Design review of the part built by this model. Coordinates are the model's own, in mm. Give positions to 0.01 mm unless a question says otherwise; leave off trailing zeros. Loops run counter-clockwise (first coordinate to the right, second up) from the corner with the lowest first, then second, coordinate; pieces in that order, holes last. Notation, with made-up numbers: (77.25, 67.5) -> (85.25, 67.5) arc R8 ccw to (85.25, 75.5) -> close; hole circle Ø10 at (-25.75, 69). An arc over 180 degrees is marked (long way). Answer in a Markdown table with one row per item. Add a question column.
(1) Consider section A-A on y = 153.5. Write out the cut boundary in (x, z), then the cut area to 3 significant figures.
(2) For pin 1 (1.2 mm diameter, centred on x = -91.5, z = 1, fed in from -Y), flat-tipped, find the tip position at first contact; note if it passes through.
(3) Consider section B-B on z = 0.7. Write out the cut boundary in (x, y), then the cut area to 3 significant figures.
(4) For line 1 (X direction, y = 152.5, z = 0.3); line 2 (X direction, y = 163, z = 0.55), list the stretches that pass through material, from the lowest coordinate up.
from build123d import *

# Parameters (mm, degrees)
RESSALTO_EXTRUS_O1_DEPTH = 2.5
FILETE1_R                = 0.1


with BuildPart() as part:
    # Esboço1 → Ressalto-extrusão1 (new body)
    with BuildSketch(Plane.XY):
        with BuildLine():
            Line((-12.454787307, 163.73471538), (-93.454787307, 163.73471538))
            ThreePointArc((-93.454787307, 163.73471538), (-95.22255426, 163.002482333), (-95.954787307, 161.23471538))
            Line((-95.954787307, 161.23471538), (-95.954787307, 152.23471538))
            ThreePointArc((-95.954787307, 152.23471538), (-95.22255426, 150.466948427), (-93.454787307, 149.73471538))
            Line((-93.454787307, 149.73471538), (-92.554787307, 149.73471538))
            Line((-92.554787307, 149.73471538), (-92.554787307, 154.73471538))
            Line((-92.554787307, 154.73471538), (-90.054787307, 154.73471538))
            Line((-90.054787307, 154.73471538), (-90.054787307, 149.73471538))
            Line((-90.054787307, 149.73471538), (-66.954787307, 149.73471538))
            Line((-66.954787307, 149.73471538), (-64.454787307, 149.73471538))
            Line((-64.454787307, 149.73471538), (-41.454787307, 149.73471538))
            Line((-41.454787307, 149.73471538), (-38.954787307, 149.73471538))
            Line((-38.954787307, 149.73471538), (-15.854787307, 149.73471538))
            Line((-15.854787307, 149.73471538), (-15.854787307, 154.73471538))
            Line((-15.854787307, 154.73471538), (-13.354787307, 154.73471538))
            Line((-13.354787307, 154.73471538), (-13.354787307, 149.73471538))
            Line((-13.354787307, 149.73471538), (-12.454787307, 149.73471538))
            ThreePointArc((-12.454787307, 149.73471538), (-10.687020354, 150.466948427), (-9.954787307, 152.23471538))
            Line((-9.954787307, 152.23471538), (-9.954787307, 161.23471538))
            ThreePointArc((-9.954787307, 161.23471538), (-10.687020354, 163.002482333), (-12.454787307, 163.73471538))
        make_face()
    extrude(amount=RESSALTO_EXTRUS_O1_DEPTH)

    # Filete1
    filete1_edges = [part.edges().sort_by_distance(p)[0] for p in [
        (-93.004787307, 149.73471538, 2.5),
        (-95.22255426, 163.002482333, 0),
        (-52.954787307, 163.73471538, 0),
        (-92.554787307, 152.23471538, 2.5),
        (-10.687020354, 163.002482333, 0),
        (-9.954787307, 156.73471538, 0),
        (-10.687020354, 150.466948427, 0),
        (-12.904787307, 149.73471538, 0),
        (-13.354787307, 152.23471538, 0),
        (-14.604787307, 154.73471538, 0),
        (-15.854787307, 152.23471538, 0),
        (-52.954787307, 149.73471538, 0),
        (-91.304787307, 154.73471538, 2.5),
        (-90.054787307, 152.23471538, 0),
        (-91.304787307, 154.73471538, 0),
        (-92.554787307, 152.23471538, 0),
        (-93.004787307, 149.73471538, 0),
        (-95.22255426, 150.466948427, 0),
        (-95.954787307, 156.73471538, 0),
        (-90.054787307, 152.23471538, 2.5),
        (-52.954787307, 149.73471538, 2.5),
        (-13.354787307, 149.73471538, 1.25),
        (-13.354787307, 154.73471538, 1.25),
        (-15.854787307, 154.73471538, 1.25),
        (-15.854787307, 149.73471538, 1.25),
        (-90.054787307, 149.73471538, 1.25),
        (-90.054787307, 154.73471538, 1.25),
        (-92.554787307, 154.73471538, 1.25),
        (-92.554787307, 149.73471538, 1.25),
        (-15.854787307, 152.23471538, 2.5),
        (-14.604787307, 154.73471538, 2.5),
        (-13.354787307, 152.23471538, 2.5),
        (-12.904787307, 149.73471538, 2.5),
        (-10.687020354, 150.466948427, 2.5),
        (-95.954787307, 156.73471538, 2.5),
        (-9.954787307, 156.73471538, 2.5),
        (-10.687020354, 163.002482333, 2.5),
        (-52.954787307, 163.73471538, 2.5),
        (-95.22255426, 163.002482333, 2.5),
        (-95.22255426, 150.466948427, 2.5),
    ]]
    fillet(filete1_edges, radius=FILETE1_R)


solid = part.part
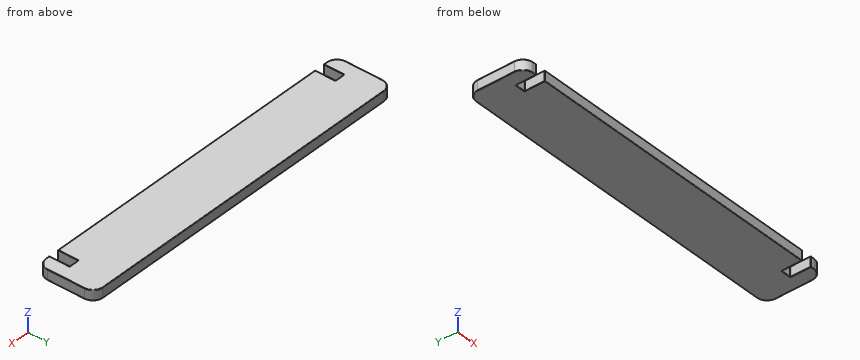
Values follow:
| question | item | result |
|---|---|---|
| 1 | outline | (-95.95, 0.1) arc R0.1 ccw to (-95.85, 0) -> (-92.65, 0) arc R0.1 ccw to (-92.55, 0.1) -> (-92.55, 2.4) arc R0.1 ccw to (-92.65, 2.5) -> (-95.85, 2.5) arc R0.1 ccw to (-95.95, 2.4) -> close; (-90.05, 0.1) arc R0.1 ccw to (-89.95, 0) -> (-15.95, 0) arc R0.1 ccw to (-15.85, 0.1) -> (-15.85, 2.4) arc R0.1 ccw to (-15.95, 2.5) -> (-89.95, 2.5) arc R0.1 ccw to (-90.05, 2.4) -> close; (-13.35, 0.1) arc R0.1 ccw to (-13.25, 0) -> (-10.05, 0) arc R0.1 ccw to (-9.95, 0.1) -> (-9.95, 2.4) arc R0.1 ccw to (-10.05, 2.5) -> (-13.25, 2.5) arc R0.1 ccw to (-13.35, 2.4) -> close |
| 1 | area | 202 mm2 |
| 2 | pin 1 | y = 154.73 |
| 3 | outline | (-95.95, 152.23) arc R2.5 ccw to (-93.45, 149.73) -> (-92.65, 149.73) arc R0.1 ccw to (-92.55, 149.83) -> (-92.55, 154.63) arc R0.1 cw to (-92.45, 154.73) -> (-90.15, 154.73) arc R0.1 cw to (-90.05, 154.63) -> (-90.05, 149.83) arc R0.1 ccw to (-89.95, 149.73) -> (-15.95, 149.73) arc R0.1 ccw to (-15.85, 149.83) -> (-15.85, 154.63) arc R0.1 cw to (-15.75, 154.73) -> (-13.45, 154.73) arc R0.1 cw to (-13.35, 154.63) -> (-13.35, 149.83) arc R0.1 ccw to (-13.25, 149.73) -> (-12.45, 149.73) arc R2.5 ccw to (-9.95, 152.23) -> (-9.95, 161.23) arc R2.5 ccw to (-12.45, 163.73) -> (-93.45, 163.73) arc R2.5 ccw to (-95.95, 161.23) -> close |
| 3 | area | 1,170 mm2 |
| 4 | line 1 | -95.95 to -92.55, -90.05 to -15.85, -13.35 to -9.95 |
| 4 | line 2 | -95.23 to -10.68 |
